Autodesk Inventor part; units mm, degrees
ref_plane "YZ Plane" through (0, 0, 0) normal (1, 0, 0) x (0, 1, 0)
ref_plane "XZ Plane" through (0, 0, 0) normal (0, 1, 0) x (-1, 0, 0)
ref_plane "XY Plane" through (0, 0, 0) normal (0, 0, 1) x (1, 0, 0)
sketch "Sketch1" plane through (0, 0, 0) normal (0, 1, 0) x (-1, 0, 0)
  line L0 (0, 0) -> (152.4, 0)
  line L1 (152.4, 0) -> (152.4, -177.8)
  line L2 (152.4, -177.8) -> (0, -177.8)
  line L3 (0, -177.8) -> (0, 0)
  dimension "d0" = 152.4
  dimension "d1" = 177.8
extrude "Extrusion1" add sketch "Sketch1" along normal blind 2.54
sketch "Sketch2" plane through (0, 2.54, 0) normal (0, 1, 0) x (1, 0, 0)
  line L0 (-152.4, 0) -> (0, 0)
  line L1 (0, 0) -> (0, 177.8)
  line L2 (0, 177.8) -> (-152.4, 177.8)
  line L3 (-152.4, 177.8) -> (-152.4, 0)
  line L4 (-146.05, 6.35) -> (-6.35, 6.35) construction
  line L5 (-6.35, 6.35) -> (-6.35, 171.45) construction
  line L6 (-6.35, 171.45) -> (-146.05, 171.45) construction
  line L7 (-146.05, 171.45) -> (-146.05, 6.35) construction
  line L8 (-146.05, 171.45) -> (-127, 171.45) construction
  line L9 (-127, 171.45) -> (-127, 6.35) construction
  line L10 (-127, 6.35) -> (-146.05, 6.35) construction
  line L11 (-146.05, 6.35) -> (-146.05, 171.45) construction
  line L12 (-76.2, 6.35) -> (-127, 6.35) construction
  line L13 (-127, 6.35) -> (-127, 171.45) construction
  line L14 (-127, 171.45) -> (-76.2, 171.45) construction
  line L15 (-76.2, 171.45) -> (-76.2, 6.35) construction
  line L16 (-25.4, 6.35) -> (-6.35, 6.35) construction
  line L17 (-6.35, 6.35) -> (-6.35, 171.45) construction
  line L18 (-6.35, 171.45) -> (-25.4, 171.45) construction
  line L19 (-25.4, 171.45) -> (-25.4, 6.35) construction
  line L20 (0, 0) -> (0, 177.8) construction
  line L21 (-152.4, 0) -> (0, 0) construction
  line L22 (0, 0) -> (0, 12.7) construction
  line L23 (0, 12.7) -> (-152.4, 12.7) construction
  line L24 (-152.4, 12.7) -> (-152.4, 0) construction
  line L25 (-152.4, 177.8) -> (0, 177.8) construction
  line L26 (0, 177.8) -> (0, 165.1) construction
  line L27 (0, 165.1) -> (-152.4, 165.1) construction
  line L28 (-152.4, 165.1) -> (-152.4, 177.8) construction
  line L29 (-146.05, 38.1) -> (-6.35, 38.1) construction
  line L30 (-6.35, 38.1) -> (-6.35, 12.7) construction
  line L31 (-6.35, 12.7) -> (-146.05, 12.7) construction
  line L32 (-146.05, 12.7) -> (-146.05, 38.1) construction
  line L33 (-146.05, 38.1) -> (-6.35, 38.1) construction
  line L34 (-6.35, 38.1) -> (-6.35, 88.9) construction
  line L35 (-6.35, 88.9) -> (-146.05, 88.9) construction
  line L36 (-146.05, 88.9) -> (-146.05, 38.1) construction
  line L37 (-6.35, 88.9) -> (-146.05, 88.9) construction
  line L38 (-146.05, 88.9) -> (-146.05, 139.7) construction
  line L39 (-146.05, 139.7) -> (-6.35, 139.7) construction
  line L40 (-6.35, 139.7) -> (-6.35, 88.9) construction
  line L41 (-146.05, 139.7) -> (-6.35, 139.7) construction
  line L42 (-6.35, 139.7) -> (-6.35, 165.1) construction
  line L43 (-6.35, 165.1) -> (-146.05, 165.1) construction
  line L44 (-146.05, 165.1) -> (-146.05, 139.7) construction
  point P0 (-146.05, 88.9)
  dimension "d4" = 6.35
  dimension "d5" = 25.4
  dimension "d6" = 25.4
  dimension "d7" = 50.8
  dimension "d8" = 12.7
  dimension "d9" = 12.7
  dimension "d10" = 25.4
  dimension "d11" = 25.4
  dimension "d12" = 76.2
hole "Hole1" at (-127, 2.54, -6.35) at (-76.2, 2.54, -6.35) at (-25.4, 2.54, -6.35) at (-127, 2.54, -171.45) at (-76.2, 2.54, -171.45) at (-25.4, 2.54, -171.45) at (-146.05, 2.54, -38.1) at (-146.05, 2.54, -88.9) at (-146.05, 2.54, -139.7) at (-6.35, 2.54, -38.1) at (-6.35, 2.54, -88.9) at (-6.35, 2.54, -139.7) direction (0, -1, 0) diameter 7.112 end through all
properties part number "090003-1"
For this review, take the finished solid that the model builds, in its own axes (mm). Give positions to 0.01 mm unless a question says otherwise; leave off trailing zeros. Write each loop counter-clockwise with the first axis right and the second up, starting at its lowest first coordinate (ties: lowest second). Pieces come first, ordered by that corner, then holes. Notation, with made-up numbers: M 3,69.25 L 20,69.25 A26 ccw 20,104.25 Z; hole C 22,-7 d1. An arc over 180 degrees is marked long. One line per item, written item: value.
1) Take a section at C-C, the plane x = -146.05. Write out the cut boundary in (y, z).
Results are:
outline: M 0,-177.8 L 2.54,-177.8 L 2.54,-143.26 L 0,-143.26 Z; M 0,-136.14 L 2.54,-136.14 L 2.54,-92.46 L 0,-92.46 Z; M 0,-85.34 L 2.54,-85.34 L 2.54,-41.66 L 0,-41.66 Z; M 0,-34.54 L 2.54,-34.54 L 2.54,0 L 0,0 Z
2) Take a section at D-D, the plane y = 1.6. Count the separate pieces of the cut face and the enclosed holes in it, then the cut area to 3 significant figures.
Results are:
separate pieces: 1
enclosed holes: 12
area: 26,600 mm²
3) Take a section at B-B, the plane z = -6.35. Write out the cut boundary in (x, y), then the cut area to 3 significant figures.
Results are:
outline: M -152.4,0 L -130.56,0 L -130.56,2.54 L -152.4,2.54 Z; M -123.44,0 L -79.76,0 L -79.76,2.54 L -123.44,2.54 Z; M -72.64,0 L -28.96,0 L -28.96,2.54 L -72.64,2.54 Z; M -21.84,0 L 0,0 L 0,2.54 L -21.84,2.54 Z
area: 333 mm²
4) Take a section at A-A, the plane x = -127. Write out the cut boundary in (y, z).
Results are:
outline: M 0,-177.8 L 2.54,-177.8 L 2.54,-175.01 L 0,-175.01 Z; M 0,-167.89 L 2.54,-167.89 L 2.54,-9.91 L 0,-9.91 Z; M 0,-2.79 L 2.54,-2.79 L 2.54,0 L 0,0 Z
5) For P1, Ø2, axis at x = -106.5, z = -150.5, coming from the -Y side, flat-tipped, find the tip position at first contact; note if it passes through.
Results are:
P1: stops at y = 0
6) For line 1 (Z direction, x = -6.35, y = 0.8); line 2 (X direction, y = 0.6, z = -6.35); line 3 (Z direction, x = -127, y = 1.7), list the stretches that pass through material, from the lowest coordinate up. Write a range as from..to.
Results are:
line 1: z = -177.8..-143.26, -136.14..-92.46, -85.34..-41.66, -34.54..0
line 2: x = -152.4..-130.56, -123.44..-79.76, -72.64..-28.96, -21.84..0
line 3: z = -177.8..-175.01, -167.89..-9.91, -2.79..0
7) The part is to be moulded in two halves that separate along X. For faces 1 (the cylindrical face through (-147.12, 1.25, -136.31)), 2 (the flat face through (-75, 0, -88)), say which applies: +X half, -X half, draft (parallel to the pull), parting line (faces both ways), or undercut.
Results are:
face 1: undercut
face 2: draft
